Input: part model. Units: mm. Frame: model coordinates. Face numbers are marked on the shaded views. A direction names the side the tool comes from. Round coordinates to 2 decimals unless told otherwise and drop trailing zeros. Write each loop counter-clockwise with the first axis right and the second up, starting at its lowest first coordinate (ties: lowest second). Pieces come first, ordered by that corner, then holes. Notation, with made-up numbers: M 33,-14 L 54,-14 A12 ccw 54,-10 Z; hole C -8.5,21.5 d4. An arc over 180 degrees is marked long. Answer as CSV lines item,"result". Start each with the question number.
```python
from build123d import *

# Parameters (mm, degrees)
SKETCH1_R           = 85
BOSS_EXTRUDE2_DEPTH = 180
SKETCH2_W           = 90
SKETCH2_H           = 90
BOSS_EXTRUDE3_DEPTH = 50
SKETCH4_R           = 65
BOSS_EXTRUDE4_DEPTH = 50
SKETCH5_R           = 85
BOSS_EXTRUDE5_DEPTH = 180
SKETCH6_W           = 90
SKETCH6_H           = 90
CUT_EXTRUDE2_DEPTH  = 50


with BuildPart() as part:
    # Sketch1 → Boss-Extrude2 (new body)
    with BuildSketch(Plane(origin=(0, 0, 0), x_dir=(1, 0, 0), z_dir=(0, 1, 0))):
        with Locations(Location((0, 0, 0), (0, 0, 90))):
            Circle(SKETCH1_R)
    extrude(amount=BOSS_EXTRUDE2_DEPTH)

    # Sketch2 → Boss-Extrude3 (add)
    with BuildSketch(Plane.XZ):
        Rectangle(SKETCH2_W, SKETCH2_H)
    extrude(amount=BOSS_EXTRUDE3_DEPTH)

    # Sketch4 → Boss-Extrude4 (add)
    with BuildSketch(Plane(origin=(0, 180, 0), x_dir=(1, 0, 0), z_dir=(0, 1, 0))):
        with Locations(Location((0, 0, 0), (0, 0, 270))):
            Circle(SKETCH4_R)
    extrude(amount=BOSS_EXTRUDE4_DEPTH)

    # Sketch5 → Boss-Extrude5 (add)
    with BuildSketch(Plane(origin=(0, 230, 0), x_dir=(1, 0, 0), z_dir=(0, 1, 0))):
        with Locations(Location((0, 0, 0), (0, 0, 90))):
            Circle(SKETCH5_R)
    extrude(amount=BOSS_EXTRUDE5_DEPTH)

    # Sketch6 → Cut-Extrude2 (cut)
    with BuildSketch(Plane(origin=(0, 410, 0), x_dir=(1, 0, 0), z_dir=(0, 1, 0))):
        Rectangle(SKETCH6_W, SKETCH6_H)
    extrude(amount=-CUT_EXTRUDE2_DEPTH, mode=Mode.SUBTRACT)


solid = part.part
```
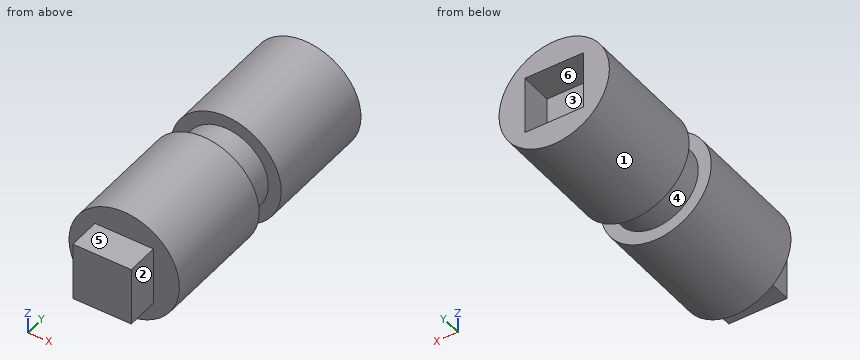
Item 1: Access query for the marked faces 4, 5 and 6. Directions: +Z, -Z, +X, -X, +Y, -Y. A direction counts if a zero-diameter tool reaches every point of the face in a straight line with its end or side. Return the directions, or none.
Item 2: Cut plane A-A, the plane z = 72.5. Return loops of the section in (x, y), plus the area to 3 significant figures.
Item 3: Cut plane D-D, the plane y = 207. Return loops of the section in (x, z).
Item 4: Line query: line 1 (Y direction, x = 76, z = -18); line 2 (Y direction, x = -56.5, z = -13.5); line 3 (Z direction, x = 1.5, y = 348). Output: solid intervals per line, ascending. Write a range as [from, to].
Item 5: Cut plane C-C, the plane z = 0. Return loops of the section in (x, y).
Item 6: Draft query along X for the marked faces 1, 2 and 3. Return one class per face: +X half, -X half, draft (parallel to the pull), parting line (faces both ways), or undercut.
Item 7: Cut plane B-B, the plane x = 0. Return loops of the section in (y, z), plus the area to 3 significant figures.
Item 8: Pin query (flat end, axial travel): pin 1 Ø4 at (x, y) = (64.5, 290) entering from -Z; pin 2 Ø2 at (y, z) = (153.5, 36) entering from -X; pin 3 Ø4 at (y, z) = (206.5, -27) entering from -X. Return the tip coordinate at first contact, or that it passes through.
Results list:
1,face 4,"none"
1,face 5,"+Z, +X, -X, -Y"
1,face 6,"+Y"
2,outline,"M -44.37,0 L 44.37,0 L 44.37,180 L -44.37,180 Z; M -44.37,230 L 44.37,230 L 44.37,410 L -44.37,410 Z"
2,area,"31,900 mm²"
3,outline,"C 0,0 d130"
4,line 1,"[0, 180], [230, 410]"
4,line 2,"[0, 410]"
4,line 3,"[-84.99, 84.99]"
5,outline,"M -85,0 L -45,0 L -45,-50 L 45,-50 L 45,0 L 85,0 L 85,180 L 65,180 L 65,230 L 85,230 L 85,410 L 45,410 L 45,360 L -45,360 L -45,410 L -85,410 L -85,230 L -65,230 L -65,180 L -85,180 Z"
6,face 1,"parting line"
6,face 2,"+X half"
6,face 3,"undercut"
7,outline,"M -50,-45 L 0,-45 L 0,-85 L 180,-85 L 180,-65 L 230,-65 L 230,-85 L 410,-85 L 410,-45 L 360,-45 L 360,45 L 410,45 L 410,85 L 230,85 L 230,65 L 180,65 L 180,85 L 0,85 L 0,45 L -50,45 Z"
7,area,"67,700 mm²"
8,pin 1,"z = -57.61"
8,pin 2,"x = -77.46"
8,pin 3,"x = -60"
